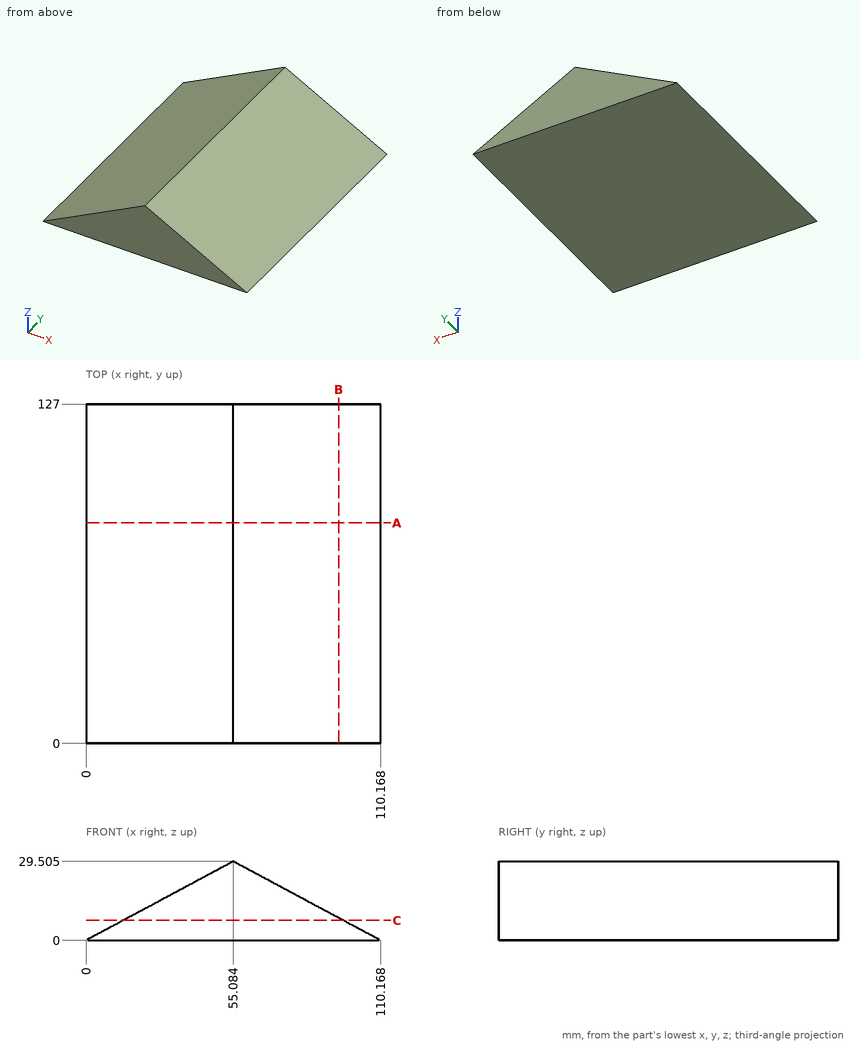
The figure shows three views and two pictorial views of one solid part (mm, origin at its lowest corner). Answer the questions. Coordinates: 2 decimals unless noted, no trailing zeros. Loops run counter-clockwise (first coordinate to the right, second up) from the corner with the lowest first, then second, coordinate; pieces in that order, holes last. Notation, with made-up numbers: M 0,68 L 50,68 A28 cw 50,92 Z; hole C -9,-5.5 d10. An arc over 180 degrees is marked long. Use CSV: the item, a comma, the result in double quotes. Start each with the question number.
(1) Find section B-B, the plane x = 94.5. Give the vertices of the cut face in (y, z), then the cut area to 3 significant figures.
(2) Find section A-A, the plane y = 82.5. Give the vertices of the cut face in (x, z) (1 decimal), then the cut area to 3 significant figures.
(3) Given pin 1 Ø5 at (x, z) = (37.5, 9) entering from -Y; pin 2 Ø10 at (y, z) = (38, 7.5) entering from +X; pin 3 Ø8 at (y, z) = (28, 7) entering from +X (1 decimal); pin 4 Ø12 at (x, z) = (81, 25.5) entering from -Y, each flat-ended and moving along its own axis, determine where each tip first touches the part or whether it passes through.
(4) Find section C-C, the plane z = 7.5. Give the vertices of the cut face in (x, y) (1 decimal), then the cut area to 3 significant figures.
(5) Consider line 1 (Z direction, x = 50.5, y = 79.5); line 2 (X direction, y = 50, z = 17.75) (1 decimal); line 3 (X direction, y = 71.5, z = 26.5) (1 decimal). Determine where each line is inside the solid, lowest interval first.
Recorded:
1,outline,"M 0,0 L 127,0 L 127,8.39 L 0,8.39 Z"
1,area,"1,070 mm^2"
2,outline,"M 0,0 L 110.2,0 L 55.1,29.5 Z"
2,area,"1,630 mm^2"
3,pin 1,"stops at y = 0"
3,pin 2,"stops at x = 105.5"
3,pin 3,"stops at x = 104.6"
3,pin 4,"passes through"
4,outline,"M 14,0 L 96.2,0 L 96.2,127 L 14,127 Z"
4,area,"10,400 mm^2"
5,line 1,"z = 0 to 27.05"
5,line 2,"x = 33.1 to 77"
5,line 3,"x = 49.5 to 60.7"
